from build123d import *

# Parameters (mm, degrees)
RESSALTO_EXTRUS_O1_DEPTH = 5
ESBO_O3_R                = 3
ESBO_O3_R_2              = 1.6
CORTE_EXTRUS_O1_DEPTH    = 10


with BuildPart() as part:
    # Esboço1 → Ressalto-extrusão1 (new body)
    with BuildSketch(Plane.XZ.offset(5)):
        with BuildLine():
            ThreePointArc((-19.691703555, 75.492649623), (-16.544693651, 74.447916667), (-17.213433323, 71.200159666))
            add(Edge.make_bspline(
                [(-17.213433323, 71.200159666), (-19.371007478, 69.977475346), (-20.225381706, 65.490339119)],
                knots=[3.520301614, 3.520301614, 3.520301614, 4.832179179, 4.832179179, 4.832179179], degree=2, weights=[1, 0.79247571, 1]))
            ThreePointArc((-20.225381706, 65.490339119), (-19.386510918, 64.613489082), (-18.509660881, 63.774618294))
            add(Edge.make_bspline(
                [(-18.509660881, 63.774618294), (-14.022524654, 64.628992522), (-12.799840334, 66.786566677)],
                knots=[4.592598781, 4.592598781, 4.592598781, 5.904476347, 5.904476347, 5.904476347], degree=2, weights=[1, 0.79247571, 1]))
            ThreePointArc((-12.799840334, 66.786566677), (-9.552083333, 67.455306349), (-8.507350377, 64.308296445))
            add(Edge.make_bspline(
                [(-8.507350377, 64.308296445), (-9.764522246, 62.170633685), (-8.260863918, 57.857472608)],
                knots=[0.37870896, 0.37870896, 0.37870896, 1.690586526, 1.690586526, 1.690586526], degree=2, weights=[1, 0.79247571, 1]))
            ThreePointArc((-8.260863918, 57.857472608), (-7.095955487, 57.517533596), (-5.917145685, 57.2294752))
            add(Edge.make_bspline(
                [(-5.917145685, 57.2294752), (-2.458358837, 60.2129531), (-2.478270232, 62.692809289)],
                knots=[4.592598781, 4.592598781, 4.592598781, 5.904476347, 5.904476347, 5.904476347], degree=2, weights=[1, 0.79247571, 1]))
            ThreePointArc((-2.478270232, 62.692809289), (0, 64.895833333), (2.478270232, 62.692809289))
            add(Edge.make_bspline(
                [(2.478270232, 62.692809289), (2.458358837, 60.2129531), (5.917145685, 57.2294752)],
                knots=[3.520301614, 3.520301614, 3.520301614, 4.832179179, 4.832179179, 4.832179179], degree=2, weights=[1, 0.79247571, 1]))
            ThreePointArc((5.917145685, 57.2294752), (7.095955487, 57.517533596), (8.260863918, 57.857472608))
            add(Edge.make_bspline(
                [(8.260863918, 57.857472608), (9.764522246, 62.170633685), (8.507350377, 64.308296445)],
                knots=[4.592598781, 4.592598781, 4.592598781, 5.904476347, 5.904476347, 5.904476347], degree=2, weights=[1, 0.79247571, 1]))
            ThreePointArc((8.507350377, 64.308296445), (9.552083333, 67.455306349), (12.799840334, 66.786566677))
            add(Edge.make_bspline(
                [(12.799840334, 66.786566677), (14.022524654, 64.628992522), (18.509660881, 63.774618294)],
                knots=[3.520301614, 3.520301614, 3.520301614, 4.832179179, 4.832179179, 4.832179179], degree=2, weights=[1, 0.79247571, 1]))
            ThreePointArc((18.509660881, 63.774618294), (19.386510918, 64.613489082), (20.225381706, 65.490339119))
            add(Edge.make_bspline(
                [(20.225381706, 65.490339119), (19.371007478, 69.977475346), (17.213433323, 71.200159666)],
                knots=[4.592598781, 4.592598781, 4.592598781, 5.904476347, 5.904476347, 5.904476347], degree=2, weights=[1, 0.79247571, 1]))
            ThreePointArc((17.213433323, 71.200159666), (16.544693651, 74.447916667), (19.691703555, 75.492649623))
            add(Edge.make_bspline(
                [(19.691703555, 75.492649623), (21.829366315, 74.235477754), (26.142527392, 75.739136082)],
                knots=[3.520301614, 3.520301614, 3.520301614, 4.832179179, 4.832179179, 4.832179179], degree=2, weights=[1, 0.79247571, 1]))
            ThreePointArc((26.142527392, 75.739136082), (26.482466404, 76.904044513), (26.7705248, 78.082854315))
            add(Edge.make_bspline(
                [(26.7705248, 78.082854315), (23.7870469, 81.541641163), (21.307190711, 81.521729768)],
                knots=[4.592598781, 4.592598781, 4.592598781, 5.904476347, 5.904476347, 5.904476347], degree=2, weights=[1, 0.79247571, 1]))
            ThreePointArc((21.307190711, 81.521729768), (19.104166667, 84), (21.307190711, 86.478270232))
            add(Edge.make_bspline(
                [(21.307190711, 86.478270232), (23.7870469, 86.458358837), (26.7705248, 89.917145685)],
                knots=[0.37870896, 0.37870896, 0.37870896, 1.690586526, 1.690586526, 1.690586526], degree=2, weights=[1, 0.79247571, 1]))
            ThreePointArc((26.7705248, 89.917145685), (26.482466404, 91.095955487), (26.142527392, 92.260863918))
            add(Edge.make_bspline(
                [(26.142527392, 92.260863918), (21.829366315, 93.764522246), (19.691703555, 92.507350377)],
                knots=[1.451006128, 1.451006128, 1.451006128, 2.762883693, 2.762883693, 2.762883693], degree=2, weights=[1, 0.79247571, 1]))
            ThreePointArc((19.691703555, 92.507350377), (16.544693651, 93.552083333), (17.213433323, 96.799840334))
            add(Edge.make_bspline(
                [(17.213433323, 96.799840334), (19.371007478, 98.022524654), (20.225381706, 102.509660881)],
                knots=[0.37870896, 0.37870896, 0.37870896, 1.690586526, 1.690586526, 1.690586526], degree=2, weights=[1, 0.79247571, 1]))
            ThreePointArc((20.225381706, 102.509660881), (19.386510918, 103.386510918), (18.509660881, 104.225381706))
            add(Edge.make_bspline(
                [(18.509660881, 104.225381706), (14.022524654, 103.371007478), (12.799840334, 101.213433323)],
                knots=[4.592598781, 4.592598781, 4.592598781, 5.904476347, 5.904476347, 5.904476347], degree=2, weights=[1, 0.79247571, 1]))
            ThreePointArc((12.799840334, 101.213433323), (9.552083333, 100.544693651), (8.507350377, 103.691703555))
            add(Edge.make_bspline(
                [(8.507350377, 103.691703555), (9.764522246, 105.829366315), (8.260863918, 110.142527392)],
                knots=[0.37870896, 0.37870896, 0.37870896, 1.690586526, 1.690586526, 1.690586526], degree=2, weights=[1, 0.79247571, 1]))
            ThreePointArc((8.260863918, 110.142527392), (7.095955487, 110.482466404), (5.917145685, 110.7705248))
            add(Edge.make_bspline(
                [(5.917145685, 110.7705248), (2.458358837, 107.7870469), (2.478270232, 105.307190711)],
                knots=[1.451006128, 1.451006128, 1.451006128, 2.762883693, 2.762883693, 2.762883693], degree=2, weights=[1, 0.79247571, 1]))
            ThreePointArc((2.478270232, 105.307190711), (0, 103.104166667), (-2.478270232, 105.307190711))
            add(Edge.make_bspline(
                [(-2.478270232, 105.307190711), (-2.458358837, 107.7870469), (-5.917145685, 110.7705248)],
                knots=[0.37870896, 0.37870896, 0.37870896, 1.690586526, 1.690586526, 1.690586526], degree=2, weights=[1, 0.79247571, 1]))
            ThreePointArc((-5.917145685, 110.7705248), (-7.095955487, 110.482466404), (-8.260863918, 110.142527392))
            add(Edge.make_bspline(
                [(-8.260863918, 110.142527392), (-9.764522246, 105.829366315), (-8.507350377, 103.691703555)],
                knots=[1.451006128, 1.451006128, 1.451006128, 2.762883693, 2.762883693, 2.762883693], degree=2, weights=[1, 0.79247571, 1]))
            ThreePointArc((-8.507350377, 103.691703555), (-9.552083333, 100.544693651), (-12.799840334, 101.213433323))
            add(Edge.make_bspline(
                [(-12.799840334, 101.213433323), (-14.022524654, 103.371007478), (-18.509660881, 104.225381706)],
                knots=[0.37870896, 0.37870896, 0.37870896, 1.690586526, 1.690586526, 1.690586526], degree=2, weights=[1, 0.79247571, 1]))
            ThreePointArc((-18.509660881, 104.225381706), (-19.386510918, 103.386510918), (-20.225381706, 102.509660881))
            add(Edge.make_bspline(
                [(-20.225381706, 102.509660881), (-19.371007478, 98.022524654), (-17.213433323, 96.799840334)],
                knots=[1.451006128, 1.451006128, 1.451006128, 2.762883693, 2.762883693, 2.762883693], degree=2, weights=[1, 0.79247571, 1]))
            ThreePointArc((-17.213433323, 96.799840334), (-16.544693651, 93.552083333), (-19.691703555, 92.507350377))
            add(Edge.make_bspline(
                [(-19.691703555, 92.507350377), (-21.829366315, 93.764522246), (-26.142527392, 92.260863918)],
                knots=[0.37870896, 0.37870896, 0.37870896, 1.690586526, 1.690586526, 1.690586526], degree=2, weights=[1, 0.79247571, 1]))
            ThreePointArc((-26.142527392, 92.260863918), (-26.482466404, 91.095955487), (-26.7705248, 89.917145685))
            add(Edge.make_bspline(
                [(-26.7705248, 89.917145685), (-23.7870469, 86.458358837), (-21.307190711, 86.478270232)],
                knots=[1.451006128, 1.451006128, 1.451006128, 2.762883693, 2.762883693, 2.762883693], degree=2, weights=[1, 0.79247571, 1]))
            ThreePointArc((-21.307190711, 86.478270232), (-19.104166667, 84), (-21.307190711, 81.521729768))
            add(Edge.make_bspline(
                [(-21.307190711, 81.521729768), (-23.7870469, 81.541641163), (-26.7705248, 78.082854315)],
                knots=[3.520301614, 3.520301614, 3.520301614, 4.832179179, 4.832179179, 4.832179179], degree=2, weights=[1, 0.79247571, 1]))
            ThreePointArc((-26.7705248, 78.082854315), (-26.482466404, 76.904044513), (-26.142527392, 75.739136082))
            add(Edge.make_bspline(
                [(-26.142527392, 75.739136082), (-21.829366315, 74.235477754), (-19.691703555, 75.492649623)],
                knots=[4.592598781, 4.592598781, 4.592598781, 5.904476347, 5.904476347, 5.904476347], degree=2, weights=[1, 0.79247571, 1]))
        make_face()
    extrude(amount=-RESSALTO_EXTRUS_O1_DEPTH)

    # Esboço3 → Corte-extrusão1 (cut)
    with BuildSketch(Plane.XZ.offset(5)):
        with Locations((0, 84)):
            Circle(ESBO_O3_R)
        with Locations((0, 92)):
            Circle(ESBO_O3_R_2)
        with Locations((0, 76)):
            Circle(ESBO_O3_R_2)
    extrude(amount=-CORTE_EXTRUS_O1_DEPTH, mode=Mode.SUBTRACT)


solid = part.part
Work out the finished part from the listing and answer in its coordinate system (mm). Round coordinates to 2 decimals unless told otherwise and drop trailing zeros. Order: outer loops, then holes, each group sorted by start corner. A loop starts at its lowest first (then second) coordinate and runs counter-clockwise, first axis right, second up. Notation, with made-up numbers: M 29,-10.75 L 64,-10.75 A14 ccw 64,4.25 Z; hole C 68.25,-19 d9. An arc over 180 degrees is marked long. One line per item, written item: value.
Q1. Find section C-C on y = -2.85. Give the number of separate pieces and of enclosed holes in the cut face, then the cut area to 3 significant figures.
Derived:
separate pieces: 1
enclosed holes: 3
area: 1,670 mm²
Q2. Straight lines are drawn through the part: line 1 (Z direction, x = 0, y = -3); line 2 (X direction, y = -4.45, z = 66); line 3 (X direction, y = -1.35, z = 76). For each, find the intervals that lie inside material, in ascending order.
Derived:
line 1: 64.9 to 74.4, 77.6 to 81, 87 to 90.4, 93.6 to 103.1
line 2: -20.12 to -13.45, -8.41 to 8.41, 13.45 to 20.12
line 3: -26.22 to -1.6, 1.6 to 26.22
Q3. Flat-ended cylindrical pins translate along their axes: pin 1 (3 mm diameter, centred on y = -3.5, z = 81.5, fed in from +X); pin 2 (3 mm diameter, centred on x = 13.5, y = -0.5, fed in from +Z); pin 3 (3 mm diameter, centred on x = -16, y = -3, fed in from -Z). Find the tip coordinate at first contact, or state that the pin passes through.
Derived:
pin 1: x = 24.75
pin 2: z = 103.04
pin 3: z = 64.01
Q4. Find section B-B on z = 84. Write down the section's boundary in (x, y), then the cut area to 3 significant figures.
Derived:
outline: M -19.1,-5 L -3,-5 L -3,0 L -19.1,0 Z; M 3,-5 L 19.1,-5 L 19.1,0 L 3,0 Z
area: 161 mm²
Q5. Find section A-A on x = 0. Write down the section's boundary in (y, z).
Derived:
outline: M -5,64.9 L 0,64.9 L 0,74.4 L -5,74.4 Z; M -5,77.6 L 0,77.6 L 0,81 L -5,81 Z; M -5,87 L 0,87 L 0,90.4 L -5,90.4 Z; M -5,93.6 L 0,93.6 L 0,103.1 L -5,103.1 Z
Q6. Find section D-D on x = 10.5. Write down the section's boundary in (y, z).
Derived:
outline: M -5,67.77 L 0,67.77 L 0,100.23 L -5,100.23 Z
Q7. Determine the mould class of faces 1 (the face through (7.11, -2.54, 110.48)), 2 (the face through (0, -5, 78)), 3 (the face through (-7.11, -2.54, 57.52)), 4 (the face through (-16.57, -2.54, 74.49)) for opening direction X: released by +X, released by -X, zero draft, split by the parting line, or undercut.
Derived:
face 1: released by +X
face 2: zero draft
face 3: released by -X
face 4: undercut
